The listing builds one solid part. Answer for the finished solid, in the listing's coordinates (mm). Face numbers are marked on the shaded views. A direction names the side the tool comes from. Coordinates: 2 decimals unless noted, no trailing zeros. Order: outer loops, then holes, each group sorted by start corner. A loop starts at its lowest first (then second) coordinate and runs counter-clockwise, first axis right, second up. Notation, with made-up numbers: (81.25, 59) -> (124.25, 59) arc R36 ccw to (124.25, 97) -> close; hole circle Ø6 at (37, -14). An arc over 180 degrees is marked (long way). Write item = value, one per line.
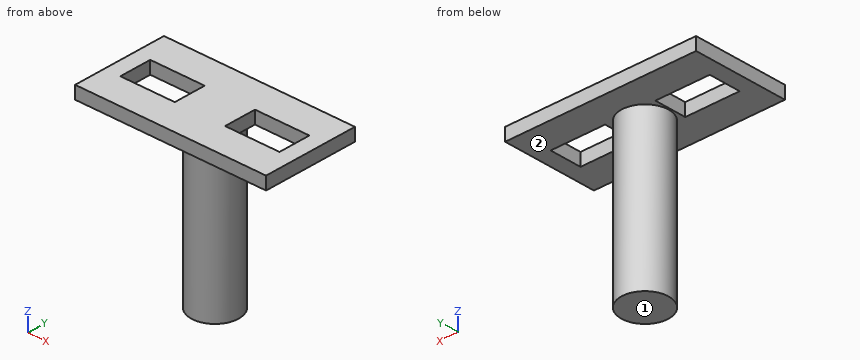
Autodesk Fusion 360 part; units mm, degrees
sketch "Sketch1" plane through (0, 0, 0) normal (0, 0, 1) x (1, 0, 0)
  line L0 (0, 0) -> (60, 0)
  line L1 (60, 0) -> (60, 30)
  line L2 (60, 30) -> (0, 30)
  line L3 (0, 30) -> (0, 0)
  circle A0 centre (30, 15) radius 7.4
  line L4 (5, 20) -> (22.0948, 20)
  line L5 (22.0948, 20) -> (22.0948, 9.9085)
  line L6 (22.0948, 9.9085) -> (5, 9.9085)
  line L7 (5, 9.9085) -> (5, 20)
  line L8 (30, 30) -> (30, 0)
  line L9 (55, 9.9085) -> (55, 20)
  line L10 (55, 20) -> (37.9052, 20)
  line L11 (37.9052, 20) -> (37.9052, 9.9085)
  line L12 (37.9052, 9.9085) -> (55, 9.9085)
  dimension "d1" = 60
  dimension "d2" = 30
  dimension "d3" = 14.8
extrude "Extrude1" add sketch "Sketch1" along normal blind 4
extrude "Extrude2" add sketch "Sketch1" against normal blind 50 contours A0 L8 | A0 L8
Q1. Each of these flat-tipped pins is pushed along its axis until it touches: pin 1 Ø2 at (x, y) = (24.5, 5.5) entering from -Z; pin 2 Ø3 at (x, z) = (38, -29.5) entering from -Y. Where does it stop, or does it pass through?
The answers:
pin_1 = 0
pin_2 = 11.46
Q2. Find the intervals of material crossed by line 1 along X through (y, z) = (14.5, -46); line 2 along Z through (x, y) = (5, 3); line 3 along Y through (x, z) = (36.5, -39), in increasing order.
The answers:
line_1 = 22.62 to 37.38
line_2 = 0 to 4
line_3 = 11.46 to 18.54
Q3. Section D-D, the plane x = 30 is taken. Give the vertices of the cut face in (y, z), plus the area to 3 significant figures.
The answers:
outline = (0, 0) -> (7.6, 0) -> (7.6, -50) -> (22.4, -50) -> (22.4, 0) -> (30, 0) -> (30, 4) -> (0, 4) -> close
area = 860 mm2
Q4. A tool of negligible diameter and unlimited length cuts with its end or side. For the marked faces 1 and 2, from which of +Z, -Z, +X, -X, +Y, -Y can it reach the whole face along a straight path? Write none if from no direction.
The answers:
face_1 = -Z, +X, -X, +Y, -Y
face_2 = -Z
Q5. Section B-B, the plane x = 13.5 is taken. Give the vertices of the cut face in (y, z).
The answers:
outline = (0, 0) -> (9.91, 0) -> (9.91, 4) -> (0, 4) -> close; (20, 0) -> (30, 0) -> (30, 4) -> (20, 4) -> close
Q6. Section A-A, the plane y = 15 is taken. Give the vertices of the cut face in (x, z), plus the area to 3 significant figures.
The answers:
outline = (0, 0) -> (5, 0) -> (5, 4) -> (0, 4) -> close; (22.09, 0) -> (22.6, 0) -> (22.6, -50) -> (37.4, -50) -> (37.4, 0) -> (37.91, 0) -> (37.91, 4) -> (22.09, 4) -> close; (55, 0) -> (60, 0) -> (60, 4) -> (55, 4) -> close
area = 843 mm2
Q7. Section C-C, the plane z = 1.5 is taken. Give the vertices of the cut face in (x, y).
The answers:
outline = (0, 0) -> (60, 0) -> (60, 30) -> (0, 30) -> close; hole (5, 9.91) -> (22.09, 9.91) -> (22.09, 20) -> (5, 20) -> close; hole (37.91, 9.91) -> (55, 9.91) -> (55, 20) -> (37.91, 20) -> close
